Source: CAD feature listing. Evaluate the final solid. Frame: model axes, mm. Give positions to 0.01 mm unless a question says otherwise; leave off trailing zeros. Order: outer loops, then holes, each group sorted by start corner. A loop starts at its lowest first (then second) coordinate and runs counter-clockwise, first axis right, second up. Notation, with made-up numbers: (15.25, 40) - (61.25, 40) arc R19 ccw to (61.25, 65) - close; hole circle Ø4 at (-12, 48.25). An arc over 180 degrees is marked (long way). One line per item, written item: value. Start each with the question number.
from build123d import *

# Parameters (mm, degrees)
BOSS_EXTRUDE1_DEPTH = 52.3875
FILLET1_R           = 12.7
FILLET2_R           = 1.27


with BuildPart() as part:
    # Sketch1 → Boss-Extrude1 (new, symmetric)
    with BuildSketch(Plane.XY):
        with BuildLine():
            ThreePointArc((-26.924, -13.081), (0, -11.938), (26.924, -13.081))
            ThreePointArc((26.924, -13.081), (40.005, 0), (26.924, 13.081))
            ThreePointArc((26.924, 13.081), (0, 11.938), (-26.924, 13.081))
            ThreePointArc((-26.924, 13.081), (-40.005, 0), (-26.924, -13.081))
        make_face()
    extrude(amount=BOSS_EXTRUDE1_DEPTH, both=True)

    # Fillet1
    # the kernel refuses this fillet: 12.7 mm, written as the material it takes off along each edge
    with BuildSketch(Plane(origin=(-26.924, 13.081, 65.711996683), x_dir=(-0.9790285886887711, -0.2037229062478567, 0), z_dir=(0, 0, -1)), Plane(origin=(-26.924, -13.081, -65.711996683), x_dir=(-0.9790285886887613, 0.20372290624790387, 0), z_dir=(0, 0, 1))) as fillet1_piece_1:
        with BuildLine():
            CenterArc((2.742517764, -12.433663076), FILLET1_R, 78.245250593, 28.210444168)
            ThreePointArc((-0.855059891, -0.253866895), (-0.427440847, -0.127233545), (0, 0))
            ThreePointArc((0, 0), (2.664899337, 0.274327031), (5.329798673, 0))
        make_face()
    extrude(amount=131.423993366, mode=Mode.SUBTRACT)
    with BuildSketch(Plane(origin=(26.924, 13.081, 65.711996683), x_dir=(-0.9965199988038926, -0.08335401600336978, 0), z_dir=(0, 0, -1))) as fillet1_piece_2:
        with BuildLine():
            CenterArc((0.909779676, -12.699987485), FILLET1_R, 90.08043566, 28.210444168)
            ThreePointArc((-5.109360575, -1.516966845), (-2.632759224, -0.495502435), (0, 0))
            ThreePointArc((0, 0), (0.445975285, -0.000313045), (0.891950569, 0))
        make_face()
    extrude(amount=131.423993366, mode=Mode.SUBTRACT)
    with BuildSketch(Plane(origin=(26.924, -13.081, -65.711996683), x_dir=(0.979028588688819, 0.20372290624762615, 0), z_dir=(0, 0, 1))) as fillet1_piece_3:
        with BuildLine():
            CenterArc((2.742517764, 12.433663076), FILLET1_R, 253.544305239, 28.210444168)
            ThreePointArc((-0.855059891, 0.253866895), (-0.427440847, 0.127233545), (0, 0))
            ThreePointArc((0, 0), (2.664899337, -0.274327031), (5.329798673, 0))
        make_face()
    extrude(amount=131.423993366, mode=Mode.SUBTRACT)

    # Fillet2
    fillet2_edges = [part.edges().sort_by_distance(p)[0] for p in [
        (40.005, 0, -52.3875),
        (40.005, 0, 52.3875),
        (-40.005, 0, -52.3875),
        (0, 11.938, -52.3875),
        (0, -11.938, -52.3875),
        (29.15115627, 12.878686287, -52.3875),
        (-29.15115627, 12.878686287, -52.3875),
        (-29.15115627, -12.878686287, -52.3875),
        (29.15115627, -12.878686287, -52.3875),
        (0, -11.938, 52.3875),
        (-40.005, 0, 52.3875),
        (0, 11.938, 52.3875),
        (29.15115627, 12.878686287, 52.3875),
        (-29.15115627, 12.878686287, 52.3875),
        (-29.15115627, -12.878686287, 52.3875),
        (29.15115627, -12.878686287, 52.3875),
    ]]
    fillet(fillet2_edges, radius=FILLET2_R)


solid = part.part
1. Ray query, L1, parallel to Y at x = -26, z = -31.5; L2, parallel to Y at x = -6, z = 13; L3, parallel to X at y = 1.25, z = -47. Return the intervals inside material, ascending.
2. Section B-B on z = -13. Return the cut outline in (x, y).
3. Contact query for flat-ended pins moving along their axis: pin 1 Ø5 at (x, z) = (15, -16.5) entering from -Y; pin 2 Ø3 at (x, z) = (-11, -30.5) entering from -Y; pin 3 Ø10 at (x, z) = (10.5, -37.5) entering from -Y. Output: stop coordinate, or through.
4. Section A-A on x = 0. Return the cut outline in (y, z).
Data:
1. L1: y = -13 to 13
1. L2: y = -11.99 to 11.99
1. L3: x = -39.95 to 39.95
2. outline: (-32.14, -12) arc R12.7 ccw to (-26.04, -13.01) arc R317.68 cw to (26.04, -13.01) arc R12.7 ccw to (32.14, -12) arc R13.08 ccw to (32.14, 12) arc R12.7 ccw to (26.04, 13.01) arc R317.68 cw to (-26.04, 13.01) arc R12.7 ccw to (-32.14, 12) arc R13.08 ccw to start
3. pin 1: stops at y = -12.42
3. pin 2: stops at y = -12.18
3. pin 3: stops at y = -12.32
4. outline: (-11.94, -51.12) arc R1.27 ccw to (-10.67, -52.39) - (10.67, -52.39) arc R1.27 ccw to (11.94, -51.12) - (11.94, 51.12) arc R1.27 ccw to (10.67, 52.39) - (-10.67, 52.39) arc R1.27 ccw to (-11.94, 51.12) - close
